Verification items for the finished model (mm, model axes). A direction names the side the tool comes from. Give positions to 0.01 mm unless a question says otherwise; leave off trailing zeros. Order: outer loops, then holes, each group sorted by start corner. A loop starts at its lowest first (then second) coordinate and runs counter-clockwise, first axis right, second up.
from build123d import *

# Parameters (mm, degrees)
F0_W    = 12.7
F0_H    = 25.4
F0_W_2  = 50.8
F0_W_3  = 19.05
F0_W_4  = 31.75
F0_H_2  = 29.9200265884
F0_H_3  = 23.518068409
F0_W_5  = 38.1
F2_SIZE = 2.54


with BuildPart() as f1:
    # F0 (on Right) → F1 (revolve)
    with BuildSketch(Plane.YZ):
        with Locations((-44.45, 31.75)):
            Rectangle(F0_W, F0_H)
        with Locations((-76.2, 31.75)):
            Rectangle(F0_W_2, F0_H)
        with Locations((41.275, 31.75)):
            Rectangle(F0_W_3, F0_H)
        with Locations((15.875, 59.4100132942)):
            Rectangle(F0_W_4, F0_H_2)
        with Locations((-44.45, 56.2090342045)):
            Rectangle(F0_W, F0_H_3)
        with Locations((-19.05, 31.75)):
            Rectangle(F0_W_5, F0_H)
        with Locations((15.875, 31.75)):
            Rectangle(F0_W_4, F0_H)
    revolve(axis=Axis((0, -50.8, 0), (0, -1, 0)))

    # F2
    f2_edges = [f1.edges().sort_by_distance(p)[0] for p in [
        (0, -101.6, -44.45),
    ]]
    chamfer(f2_edges, length=F2_SIZE)


solid = f1.part
(1) Section check C-C, the plane y = 41.5. Enter the section's corners in (x, z), then the cut area to 3 significant figures.
Solved:
outline: circle Ø88.9 at (0, 0); hole circle Ø38.1 at (0, 0)
area: 5,070 mm2
(2) Release check for a two-part mould opening along Y. For faces 6 (the flat face through (32, 0, -32)), 7 (the cylindrical face through (11.59, -24.33, -15.12)), 8 (the flat face through (19, 50.8, -9)) record: pulls with the +Y half, pulls with the -Y half, needs draft (parallel to the pull), parting line crosses it, or undercut.
Solved:
face 6: undercut
face 7: needs draft
face 8: pulls with the +Y half
(3) Set-up check for faces 1 (the cylindrical face through (72.6, 16.1, -16.12)), 2 (the flat face through (18, -101.6, -9)), 3 (the cylindrical face through (-20.42, -44.36, 64.83)), 4 (the flat face through (44, -38.1, -14)), 5 (the flat face through (32, 31.75, -32)): record each of +Z, -Z, +X, -X, +Y, -Y from which the full face is reachable in a straight line by a thin tool's end or side.
Solved:
face 1: +Y, -Y
face 2: +Z, -Z, +X, -X, -Y
face 3: -Y
face 4: none
face 5: +Y
(4) Scan lines: line 1 (Z direction, x = 0, y = -30.5); line 2 (Y direction, x = 60, z = -16.5); line 3 (X direction, y = -48, z = 0). Record each from-to range of solid material in increasing order.
Solved:
line 1: z = -44.45 to -19.05, 19.05 to 44.45
line 2: y = -50.8 to -38.1, 0 to 31.75
line 3: x = -67.97 to -19.05, 19.05 to 67.97
(5) Section check D-D, the plane z = -50. Enter the section's corners in (x, y), then the cut area to 3 significant figures.
Solved:
outline: (-55.05, 0) - (55.05, 0) - (55.05, 31.75) - (-55.05, 31.75) - close; (-46.04, -50.8) - (46.04, -50.8) - (46.04, -38.1) - (-46.04, -38.1) - close
area: 4,670 mm2
(6) Section check A-A, the plane x = 0. Enter the section's corners in (y, z), then the cut area to 3 significant figures.
Solved:
outline: (-101.6, -41.91) - (-99.06, -44.45) - (-50.8, -44.45) - (-50.8, -67.97) - (-38.1, -67.97) - (-38.1, -44.45) - (0, -44.45) - (0, -74.37) - (31.75, -74.37) - (31.75, -44.45) - (50.8, -44.45) - (50.8, -19.05) - (-101.6, -19.05) - close; (-101.6, 19.05) - (50.8, 19.05) - (50.8, 44.45) - (31.75, 44.45) - (31.75, 74.37) - (0, 74.37) - (0, 44.45) - (-38.1, 44.45) - (-38.1, 67.97) - (-50.8, 67.97) - (-50.8, 44.45) - (-99.06, 44.45) - (-101.6, 41.91) - close
area: 10,200 mm2
(7) Section check B-B, the plane z = 0. Enter the section's corners in (x, y), then the cut area to 3 significant figures.
Solved:
outline: (-74.37, 0) - (-44.45, 0) - (-44.45, -38.1) - (-67.97, -38.1) - (-67.97, -50.8) - (-44.45, -50.8) - (-44.45, -99.06) - (-41.91, -101.6) - (-19.05, -101.6) - (-19.05, 50.8) - (-44.45, 50.8) - (-44.45, 31.75) - (-74.37, 31.75) - close; (19.05, -101.6) - (41.91, -101.6) - (44.45, -99.06) - (44.45, -50.8) - (67.97, -50.8) - (67.97, -38.1) - (44.45, -38.1) - (44.45, 0) - (74.37, 0) - (74.37, 31.75) - (44.45, 31.75) - (44.45, 50.8) - (19.05, 50.8) - close
area: 10,200 mm2
(8) Go/stop test with flat-tipped pins: pin 1 (8 mm diameter, centred on y = -64.5, z = -40, fed in from -X); pin 2 (12 mm diameter, centred on x = 5, y = -74.5, fed in from +Z); pin 3 (12 mm diameter, centred on x = 46.5, z = 30, fed in from -Y). Record where each tip stops, or that it passes through.
Solved:
pin 1: stops at x = -26.07
pin 2: stops at z = 44.45
pin 3: stops at y = -50.8
